```python
from build123d import *

# Parameters (mm, degrees)
SKETCH1_R           = 6
SKETCH1_R_2         = 1.7
BOSS_EXTRUDE1_DEPTH = 3
SKETCH2_R           = 20
SKETCH2_R_2         = 6
SKETCH2_R_3         = 1.7
BOSS_EXTRUDE2_DEPTH = 2
SKETCH3_R           = 12
SKETCH3_R_2         = 6
BOSS_EXTRUDE3_DEPTH = 2
SKETCH4_R           = 4.5
SKETCH4_R_2         = 1.7
BOSS_EXTRUDE4_DEPTH = 5
SKETCH5_R           = 4.5
SKETCH5_R_2         = 1.7
BOSS_EXTRUDE5_DEPTH = 5
SKETCH6_R           = 4.5
SKETCH6_R_2         = 1.7
BOSS_EXTRUDE6_DEPTH = 5
SKETCH7_R           = 4.5
SKETCH7_R_2         = 1.7
BOSS_EXTRUDE7_DEPTH = 5
SKETCH8_R           = 8.05
CUT_EXTRUDE1_DEPTH  = 4.5
SKETCH9_R           = 3.2
CUT_EXTRUDE2_DEPTH  = 3.2


with BuildPart() as part:
    # Sketch1 → Boss-Extrude1 (new body)
    with BuildSketch(Plane.XY.offset(328.5)):
        with BuildLine():
            Line((277.006534343, 300.548212638), (273.908821488, 170.622068635))
            ThreePointArc((273.908821488, 170.622068635), (300, 143.901406829), (326.091178512, 170.622068635))
            Line((326.091178512, 170.622068635), (322.993465657, 300.548212638))
            ThreePointArc((322.993465657, 300.548212638), (300, 323), (277.006534343, 300.548212638))
        make_face()
        with Locations((300, 300)):
            Circle(SKETCH1_R, mode=Mode.SUBTRACT)
        with Locations((300, 170)):
            Circle(SKETCH1_R, mode=Mode.SUBTRACT)
        with Locations((312.124355653, 307)):
            Circle(SKETCH1_R_2, mode=Mode.SUBTRACT)
        with Locations((287.875644347, 307)):
            Circle(SKETCH1_R_2, mode=Mode.SUBTRACT)
        with Locations((300, 286)):
            Circle(SKETCH1_R_2, mode=Mode.SUBTRACT)
        with BuildLine():
            Line((305, 258.3), (314, 258.3))
            ThreePointArc((314, 258.3), (315.7, 260), (314, 261.7))
            Line((314, 261.7), (305, 261.7))
            ThreePointArc((305, 261.7), (303.3, 260), (305, 258.3))
        make_face(mode=Mode.SUBTRACT)
        with BuildLine():
            Line((294.661250685, 252.292425307), (293.257422469, 237.959091974))
            ThreePointArc((293.257422469, 237.959091974), (294.02083171, 235.651384543), (296.243136361, 234.666666667))
            Line((296.243136361, 234.666666667), (303.756863639, 234.666666667))
            ThreePointArc((303.756863639, 234.666666667), (305.97916829, 235.651384543), (306.742577531, 237.959091974))
            Line((306.742577531, 237.959091974), (305.338749315, 252.292425307))
            ThreePointArc((305.338749315, 252.292425307), (304.368317547, 254.222304651), (302.353035423, 255))
            Line((302.353035423, 255), (297.646964577, 255))
            ThreePointArc((297.646964577, 255), (295.631682453, 254.222304651), (294.661250685, 252.292425307))
        make_face(mode=Mode.SUBTRACT)
        with BuildLine():
            Line((292.180065932, 226.959091974), (290.776237716, 212.625758641))
            ThreePointArc((290.776237716, 212.625758641), (291.539646956, 210.318051209), (293.761951607, 209.333333333))
            Line((293.761951607, 209.333333333), (306.238048393, 209.333333333))
            ThreePointArc((306.238048393, 209.333333333), (308.460353044, 210.318051209), (309.223762284, 212.625758641))
            Line((309.223762284, 212.625758641), (307.819934068, 226.959091974))
            ThreePointArc((307.819934068, 226.959091974), (306.849502301, 228.888971317), (304.834220177, 229.666666667))
            Line((304.834220177, 229.666666667), (295.165779823, 229.666666667))
            ThreePointArc((295.165779823, 229.666666667), (293.150497699, 228.888971317), (292.180065932, 226.959091974))
        make_face(mode=Mode.SUBTRACT)
        with BuildLine():
            Line((289.698881178, 201.625758641), (288.295052962, 187.292425307))
            ThreePointArc((288.295052962, 187.292425307), (289.058462202, 184.984717876), (291.280766853, 184))
            Line((291.280766853, 184), (308.719233147, 184))
            ThreePointArc((308.719233147, 184), (310.941537798, 184.984717876), (311.704947038, 187.292425307))
            Line((311.704947038, 187.292425307), (310.301118822, 201.625758641))
            ThreePointArc((310.301118822, 201.625758641), (309.330687055, 203.555637984), (307.315404931, 204.333333333))
            Line((307.315404931, 204.333333333), (292.684595069, 204.333333333))
            ThreePointArc((292.684595069, 204.333333333), (290.669312945, 203.555637984), (289.698881178, 201.625758641))
        make_face(mode=Mode.SUBTRACT)
    extrude(amount=BOSS_EXTRUDE1_DEPTH)

    # Sketch2 → Boss-Extrude2 (add)
    with BuildSketch(Plane.XY.offset(331.5)):
        with Locations((300, 300)):
            Circle(SKETCH2_R)
        with Locations((300, 300)):
            Circle(SKETCH2_R_2, mode=Mode.SUBTRACT)
        with Locations((312.124355653, 307)):
            Circle(SKETCH2_R_3, mode=Mode.SUBTRACT)
        with Locations((287.875644347, 307)):
            Circle(SKETCH2_R_3, mode=Mode.SUBTRACT)
        with Locations((300, 286)):
            Circle(SKETCH2_R_3, mode=Mode.SUBTRACT)
    extrude(amount=BOSS_EXTRUDE2_DEPTH)

    # Sketch3 → Boss-Extrude3 (add)
    with BuildSketch(Plane.XY.offset(331.5)):
        with Locations((300, 170)):
            Circle(SKETCH3_R)
        with Locations((300, 170)):
            Circle(SKETCH3_R_2, mode=Mode.SUBTRACT)
    extrude(amount=BOSS_EXTRUDE3_DEPTH)

    # Sketch4 → Boss-Extrude4 (add)
    with BuildSketch(Plane.XY.offset(328.5)):
        with Locations(Location((273.593173433, 220, 0), (0, 0, 288.004143267))):
            Circle(SKETCH4_R)
        with Locations(Location((273.593173433, 220, 0), (0, 0, 330.029047181))):
            Circle(SKETCH4_R_2, mode=Mode.SUBTRACT)
    extrude(amount=BOSS_EXTRUDE4_DEPTH)

    # Sketch5 → Boss-Extrude5 (add)
    with BuildSketch(Plane.XY.offset(328.5)):
        with Locations(Location((326.406826567, 220, 0), (0, 0, 110.735729818))):
            Circle(SKETCH5_R)
        with Locations(Location((326.406826567, 220, 0), (0, 0, 152.760633732))):
            Circle(SKETCH5_R_2, mode=Mode.SUBTRACT)
    extrude(amount=BOSS_EXTRUDE5_DEPTH)

    # Sketch6 → Boss-Extrude6 (add)
    with BuildSketch(Plane.XY.offset(328.5)):
        with Locations(Location((271.401406829, 170, 0), (0, 0, 55.009544434))):
            Circle(SKETCH6_R)
        with Locations((271.401406829, 170)):
            Circle(SKETCH6_R_2, mode=Mode.SUBTRACT)
    extrude(amount=BOSS_EXTRUDE6_DEPTH)

    # Sketch7 → Boss-Extrude7 (add)
    with BuildSketch(Plane.XY.offset(328.5)):
        with Locations(Location((328.598593171, 170, 0), (0, 0, 232.414236235))):
            Circle(SKETCH7_R)
        with Locations((328.598593171, 170)):
            Circle(SKETCH7_R_2, mode=Mode.SUBTRACT)
    extrude(amount=BOSS_EXTRUDE7_DEPTH)

    # Sketch8 → Cut-Extrude1 (cut)
    with BuildSketch(Plane.XY.offset(329)):
        with Locations((300, 300)):
            Circle(SKETCH8_R)
        with Locations((300, 170)):
            Circle(SKETCH8_R)
    extrude(amount=CUT_EXTRUDE1_DEPTH, mode=Mode.SUBTRACT)

    # Sketch9 → Cut-Extrude2 (cut)
    with BuildSketch(Plane.XY.offset(328.5)):
        with Locations((312.124355653, 307)):
            Circle(SKETCH9_R)
        with Locations((287.875644347, 307)):
            Circle(SKETCH9_R)
        with Locations((300, 286)):
            Circle(SKETCH9_R)
    extrude(amount=CUT_EXTRUDE2_DEPTH, mode=Mode.SUBTRACT)


solid = part.part
```
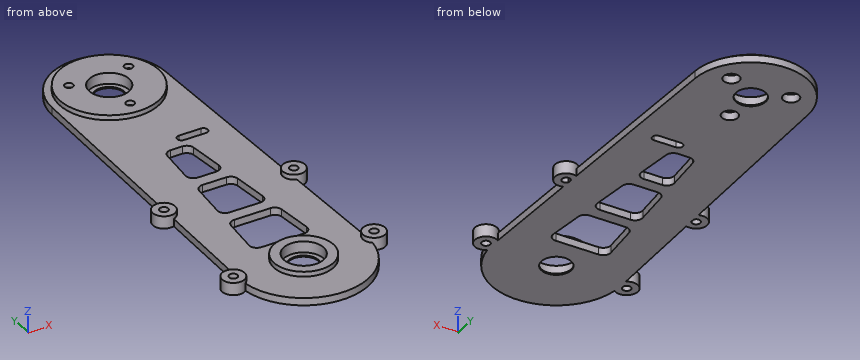
Geometry: final body of the model. Coordinates: model frame, mm. Round coordinates to 2 decimals unless told otherwise and drop trailing zeros. Write each loop counter-clockwise with the first axis right and the second up, starting at its lowest first coordinate (ties: lowest second). Pieces come first, ordered by that corner, then holes.
Item 1: Material intervals for L1, parallel to X at y = 307, z = 329.4; L2, parallel to Y at x = 312, z = 330.7; L3, parallel to Y at x = 325, z = 331.75, sorted ascending.
Item 2: Pin query (flat end, axial travel): P1, Ø8, axis at x = 300, y = 173.5, coming from the +Z side; P2, Ø1.9, axis at x = 288, y = 307.5, coming from the -Z side; P3, Ø3, axis at x = 300.5, y = 286, coming from the -Z side; P4, Ø3, axis at x = 321, z = 331.5, coming from the +Y side. Return the tip coordinate at first contact, or that it passes through.
Item 3: Section query B-B (y = 260). Return loops of the section in (x, z), plus the area to 3 significant figures.
Item 4: Section query A-A (y = 170). Return loops of the section in (x, z).
Item 5: Section query C-C (z = 329.9). Give the number of separate pieces and of enclosed holes in the cut face, plus the area to 3 significant figures.
Completed:
1. L1: x = 278.09 to 284.68, 291.08 to 296.02, 303.98 to 308.92, 315.32 to 321.91
1. L2: y = 146.82 to 258.3, 261.7 to 303.8, 310.2 to 319.62
1. L3: y = 167.3 to 172.7, 215.73 to 219.05, 220.95 to 224.27
2. P1: stops at z = 329
2. P2: passes through
2. P3: stops at z = 331.7
2. P4: stops at y = 312.2
3. outline: (276.04, 328.5) - (303.3, 328.5) - (303.3, 331.5) - (276.04, 331.5) - close; (315.7, 328.5) - (323.96, 328.5) - (323.96, 331.5) - (315.7, 331.5) - close
3. area: 107 mm2
4. outline: (266.9, 328.5) - (269.7, 328.5) - (269.7, 333.5) - (266.9, 333.5) - close; (273.1, 328.5) - (294, 328.5) - (294, 329) - (291.95, 329) - (291.95, 333.5) - (288, 333.5) - (288, 331.5) - (275.9, 331.5) - (275.9, 333.5) - (273.1, 333.5) - close; (306, 328.5) - (326.9, 328.5) - (326.9, 333.5) - (324.1, 333.5) - (324.1, 331.5) - (312, 331.5) - (312, 333.5) - (308.05, 333.5) - (308.05, 329) - (306, 329) - close; (330.3, 328.5) - (333.1, 328.5) - (333.1, 333.5) - (330.3, 333.5) - close
5. separate pieces: 1
5. enclosed holes: 13
5. area: 6,880 mm2
